Design review of the part built by this model. Coordinates are the model's own, in mm. A direction names the side the tool comes from. Coordinates: 2 decimals unless noted, no trailing zeros. Write each loop counter-clockwise with the first axis right and the second up, starting at its lowest first coordinate (ties: lowest second). Pieces come first, ordered by that corner, then holes. Notation, with made-up numbers: (11, -15.5) -> (18, -15.5) arc R14 cw to (18, 2.5) -> close; hole circle Ø7 at (-34, -37). An arc over 180 degrees is marked (long way). Answer in a Markdown table with one row per item. Add a question column.
Item 1: Draft analysis for pull direction X (two halves, no side actions). For faces 1 (the face through (0, -2, 19)), 2 (the face through (3.13, 130.15, 19.81)), 3 (the face through (20.886, 123.126, 3.131)), state which applies: released by +X, released by -X, zero draft, split by the parting line, or undercut.
Item 2: Clearance check with flat-ended pins moving along their axes: P1, Ø2, axis at x = 28, y = -4, coming from the -Z side; P2, Ø1.5, axis at y = -118.5, z = 10.5, coming from the +X side; P3, Ø2, axis at x = 16, y = 16.5, coming from the +Z side. State where each tip first meets the part, or that it passes through.
Item 3: Take a section at A-A, the plane y = 127. Write out the cut boundary in (x, z), and give its area (3 significant figures).
Item 4: Take a section at B-B, the plane x = 35. Write out the cut boundary in (y, z).
Item 5: Take a section at C-C, the plane y = -80. Write out the cut boundary in (x, z), and give its area (3 significant figures).
Item 6: For faces 4 (the face through (23.175, -129.415, 3.131)), 5 (the face through (6.35, -2, 22)), list the 3-axis set-ups (+Z, -Z, +X, -X, +Y, -Y) from which the entire face can be reached by the end or side of a thin tool; tool diameter is ignored.
Item 7: To check wall thickness, follow line 1 (Z direction, x = 2, y = 127); line 2 (X direction, y = 62.5, z = 32.5). State the ranges of each line that lie inside material, in increasing order.
Item 8: Take a section at D-D, the plane z = 35.5. Write out the cut boundary in (x, y), and give its area (3 significant figures).
from build123d import *

# Parameters (mm, degrees)
F1_DEPTH = 152.4
F3_D     = 7.9375
F5_D     = 7.9375


with BuildPart() as f1:
    # F0 (on Front) → F1 (new body, symmetric)
    with BuildSketch(Plane.XZ):
        Polygon((0, 38.1), (0, 0), (38.1, 0), (38.1, 6.35), (6.35, 6.35), (6.35, 38.1), align=None)
    extrude(amount=F1_DEPTH, both=True)

    # F3 (through all)
    with Locations(Plane.XY.offset(6.35)):
        with Locations((20.025469, -127), (20.025469, 76.2), (20.025469, 127)):
            Hole(F3_D / 2)

    # F5 (through all)
    with Locations(Plane.YZ.offset(6.35)):
        with Locations((-127, 22.225), (76.2, 22.225), (127, 22.225)):
            Hole(F5_D / 2)


solid = f1.part
Answers:
| question | item | result |
|---|---|---|
| 1 | face 1 | released by -X |
| 1 | face 2 | zero draft |
| 1 | face 3 | undercut |
| 2 | P1 | stops at z = 0 |
| 2 | P2 | stops at x = 6.35 |
| 2 | P3 | stops at z = 6.35 |
| 3 | outline | (0, 0) -> (16.06, 0) -> (16.06, 6.35) -> (6.35, 6.35) -> (6.35, 18.26) -> (0, 18.26) -> close; (0, 26.19) -> (6.35, 26.19) -> (6.35, 38.1) -> (0, 38.1) -> close; (23.99, 0) -> (38.1, 0) -> (38.1, 6.35) -> (23.99, 6.35) -> close |
| 3 | area | 343 mm^2 |
| 4 | outline | (-152.4, 0) -> (152.4, 0) -> (152.4, 6.35) -> (-152.4, 6.35) -> close |
| 5 | outline | (0, 0) -> (38.1, 0) -> (38.1, 6.35) -> (6.35, 6.35) -> (6.35, 38.1) -> (0, 38.1) -> close |
| 5 | area | 444 mm^2 |
| 6 | face 4 | +Z, -Z |
| 6 | face 5 | +Z, +X, +Y, -Y |
| 7 | line 1 | z = 0 to 18.26, 26.19 to 38.1 |
| 7 | line 2 | x = 0 to 6.35 |
| 8 | outline | (0, -152.4) -> (6.35, -152.4) -> (6.35, 152.4) -> (0, 152.4) -> close |
| 8 | area | 1,940 mm^2 |
